```python
from build123d import *

# Parameters (mm, degrees)
SKETCH_1_R                = 3.5
SKETCH_1_R_2              = 4.5
SKETCH_1_R_3              = 1.5
EXTRUDE_1_DEPTH           = 10
HOLE_WIZARD_1_D           = 6.6
HOLE_WIZARD_1_DEPTH       = 18
HOLE_WIZARD_1_CBORE_D     = 11
HOLE_WIZARD_1_CBORE_DEPTH = 6.8
HOLE_WIZARD_1_TIP         = 1.982840043


with BuildPart() as part:
    # 草图1 → 凸台-拉伸1 (new body)
    with BuildSketch(Plane.XY):
        Polygon((-270, 180), (270, 180), (280, 170), (280, -170), (270, -180), (-270, -180), (-280, -170), (-280, 170), align=None)
        with Locations((-256, 140)):
            Circle(SKETCH_1_R, mode=Mode.SUBTRACT)
        with Locations((-224, 140)):
            Circle(SKETCH_1_R, mode=Mode.SUBTRACT)
        with Locations((-256, 104)):
            Circle(SKETCH_1_R, mode=Mode.SUBTRACT)
        with Locations((-224, 104)):
            Circle(SKETCH_1_R, mode=Mode.SUBTRACT)
        with Locations((256, 104)):
            Circle(SKETCH_1_R, mode=Mode.SUBTRACT)
        with Locations((224, 104)):
            Circle(SKETCH_1_R, mode=Mode.SUBTRACT)
        with Locations((224, 140)):
            Circle(SKETCH_1_R, mode=Mode.SUBTRACT)
        with Locations((256, 140)):
            Circle(SKETCH_1_R, mode=Mode.SUBTRACT)
        with Locations((-220, -130)):
            Circle(SKETCH_1_R_2, mode=Mode.SUBTRACT)
        with Locations((-100, -130)):
            Circle(SKETCH_1_R_2, mode=Mode.SUBTRACT)
        with Locations((20, -130)):
            Circle(SKETCH_1_R_2, mode=Mode.SUBTRACT)
        with Locations((140, -130)):
            Circle(SKETCH_1_R_2, mode=Mode.SUBTRACT)
        with Locations((260, -130)):
            Circle(SKETCH_1_R_2, mode=Mode.SUBTRACT)
        with Locations((-100, -170)):
            Circle(SKETCH_1_R_2, mode=Mode.SUBTRACT)
        with Locations((20, -170)):
            Circle(SKETCH_1_R_2, mode=Mode.SUBTRACT)
        with Locations((140, -170)):
            Circle(SKETCH_1_R_2, mode=Mode.SUBTRACT)
        with Locations((260, -170)):
            Circle(SKETCH_1_R_2, mode=Mode.SUBTRACT)
        with Locations((-220, -170)):
            Circle(SKETCH_1_R_2, mode=Mode.SUBTRACT)
        with Locations((-25, 90)):
            Circle(SKETCH_1_R_3, mode=Mode.SUBTRACT)
        with Locations((-256, 45)):
            Circle(SKETCH_1_R, mode=Mode.SUBTRACT)
        with Locations((-224, 45)):
            Circle(SKETCH_1_R, mode=Mode.SUBTRACT)
        with Locations((-25, 75)):
            Circle(SKETCH_1_R_3, mode=Mode.SUBTRACT)
        with Locations((-25, 60)):
            Circle(SKETCH_1_R_3, mode=Mode.SUBTRACT)
        with Locations((-256, 9)):
            Circle(SKETCH_1_R, mode=Mode.SUBTRACT)
        with Locations((-224, 9)):
            Circle(SKETCH_1_R, mode=Mode.SUBTRACT)
        with Locations((224, 45)):
            Circle(SKETCH_1_R, mode=Mode.SUBTRACT)
        with Locations((256, 45)):
            Circle(SKETCH_1_R, mode=Mode.SUBTRACT)
        with Locations((224, 9)):
            Circle(SKETCH_1_R, mode=Mode.SUBTRACT)
        with Locations((256, 9)):
            Circle(SKETCH_1_R, mode=Mode.SUBTRACT)
        with BuildLine():
            Line((-165, 120), (-55, 120))
            ThreePointArc((-55, 120), (-47.928932188, 117.071067812), (-45, 110))
            Line((-45, 110), (-45, -110))
            ThreePointArc((-45, -110), (-47.928932188, -117.071067812), (-55, -120))
            Line((-55, -120), (-165, -120))
            ThreePointArc((-165, -120), (-172.071067812, -117.071067812), (-175, -110))
            Line((-175, -110), (-175, 110))
            ThreePointArc((-175, 110), (-172.071067812, 117.071067812), (-165, 120))
        make_face(mode=Mode.SUBTRACT)
        with BuildLine():
            Line((165, -120), (55, -120))
            ThreePointArc((55, -120), (47.928932188, -117.071067812), (45, -110))
            Line((45, -110), (45, 110))
            ThreePointArc((45, 110), (47.928932188, 117.071067812), (55, 120))
            Line((55, 120), (165, 120))
            ThreePointArc((165, 120), (172.071067812, 117.071067812), (175, 110))
            Line((175, 110), (175, -110))
            ThreePointArc((175, -110), (172.071067812, -117.071067812), (165, -120))
        make_face(mode=Mode.SUBTRACT)
    extrude(amount=EXTRUDE_1_DEPTH)

    # 打孔尺寸(%根据)内六角圆柱头螺钉的类型1
    with Locations(Plane(origin=(-256, 9, 0), x_dir=(-1, 0, 0), z_dir=(0, 0, -1))):
        with Locations((0, 0), (-480, 131), (-512, 131), (-512, 95), (-480, 95), (-512, 36), (-480, 36), (-512, 0), (-480, 0), (-231, 81), (-231, 66), (-231, 51), (-32, 131), (-32, 95), (0, 95), (0, 131), (-32, 36), (0, 36), (-32, 0)):
            CounterBoreHole(HOLE_WIZARD_1_D / 2, HOLE_WIZARD_1_CBORE_D / 2, HOLE_WIZARD_1_CBORE_DEPTH, depth=HOLE_WIZARD_1_DEPTH)
            with Locations((0, 0, -(HOLE_WIZARD_1_DEPTH + HOLE_WIZARD_1_TIP / 2))):  # 118° drill point
                Cone(0, HOLE_WIZARD_1_D / 2, HOLE_WIZARD_1_TIP, mode=Mode.SUBTRACT)


solid = part.part
```
Here's how the part is built. I have some questions about the finished solid (model axes, mm). A direction names the side the tool comes from. Round coordinates to 2 decimals unless told otherwise and drop trailing zeros. Order: outer loops, then holes, each group sorted by start corner. A loop starts at its lowest first (then second) coordinate and runs counter-clockwise, first axis right, second up. Notation, with made-up numbers: (-0.75, -23) -> (9.25, -23) arc R28 cw to (9.25, -5) -> close; hole circle Ø7 at (86.25, -14). An arc over 180 degrees is marked (long way). Use a Markdown table: item, result. Add a question column.
(1) If we mould it in two halves opening along X, with no side actions, what happens to faces 4 (the face through (-45, 2, 5)), 5 (the face through (-275, 175, 5)), 6 (the face through (4, -180, 5))? For each: released by +X, released by -X, zero draft, split by the parting line, or undercut.
(2) I need wall thicknesses on line 1 along Y through (x, z) = (-25, 2.25); line 2 along Y through (x, z) = (224, 1.75); line 3 along Y through (x, z) = (-25, 7.5). Which ranges of each line are inside material? Lowest first, please.
(3) For faces 1 (the face through (275, -175, 5)), 2 (the face through (172.15, -116.99, 4.93)), 3 (the face through (250.92, 6.89, 3.35)), which set-ups out of +Z, -Z, +X, -X, +Y, -Y let a thin tool reach every point of the face, with its end or its side?
(4) Suppose I cut it at A-A, the plane x = 88. Please give me the cut outline in (y, z), and give its area (3 significant figures).
(5) Suppose I cut it at C-C, the plane z = 8.5. Count the separate pieces of the cut face and the enclosed holes in it, and give its area (3 significant figures).
(6) Suppose I cut it at B-B, the plane y = -43. Please give me the cut outline in (x, z).
(7) For pin 1 Ø10 at (x, y) = (-256, 9) entering from +Z; pin 2 Ø5.5 at (x, y) = (-226, 141.5) entering from -Z; pin 3 Ø6.5 at (x, y) = (-224, 140) entering from -Z, each with a flat end and sliding along its axis, tell me the tip position at first contact or that it passes through.
Verdict:
| question | item | result |
|---|---|---|
| 1 | face 4 | undercut |
| 1 | face 5 | released by -X |
| 1 | face 6 | zero draft |
| 2 | line 1 | -180 to 54.5, 65.5 to 69.5, 80.5 to 84.5, 95.5 to 180 |
| 2 | line 2 | -180 to 3.5, 14.5 to 39.5, 50.5 to 98.5, 109.5 to 134.5, 145.5 to 180 |
| 2 | line 3 | -180 to 56.7, 63.3 to 71.7, 78.3 to 86.7, 93.3 to 180 |
| 3 | face 1 | +Z, -Z, +X, -Y |
| 3 | face 2 | +Z, -Z |
| 3 | face 3 | -Z |
| 4 | outline | (-180, 0) -> (-120, 0) -> (-120, 10) -> (-180, 10) -> close; (120, 0) -> (180, 0) -> (180, 10) -> (120, 10) -> close |
| 4 | area | 1,200 mm2 |
| 5 | separate pieces | 1 |
| 5 | enclosed holes | 31 |
| 5 | area | 138,000 mm2 |
| 6 | outline | (-280, 0) -> (-175, 0) -> (-175, 10) -> (-280, 10) -> close; (-45, 0) -> (45, 0) -> (45, 10) -> (-45, 10) -> close; (175, 0) -> (280, 0) -> (280, 10) -> (175, 10) -> close |
| 7 | pin 1 | z = 10 |
| 7 | pin 2 | z = 6.8 |
| 7 | pin 3 | through |
